The figure shows three views and two pictorial views of one solid part (mm, origin at its lowest corner). Answer the questions. Give positions to 0.01 mm unless a question says otherwise; leave off trailing zeros. Loops run counter-clockwise (first coordinate to the right, second up) from the corner with the lowest first, then second, coordinate; pieces in that order, holes last. Notation, with made-up numbers: M 64,-37 L 72,-37 A22 ccw 72,-11 Z; hole C -4,86.5 d5. An arc over 180 degrees is marked long. Answer in a Markdown table with one row per item. Add a question column.
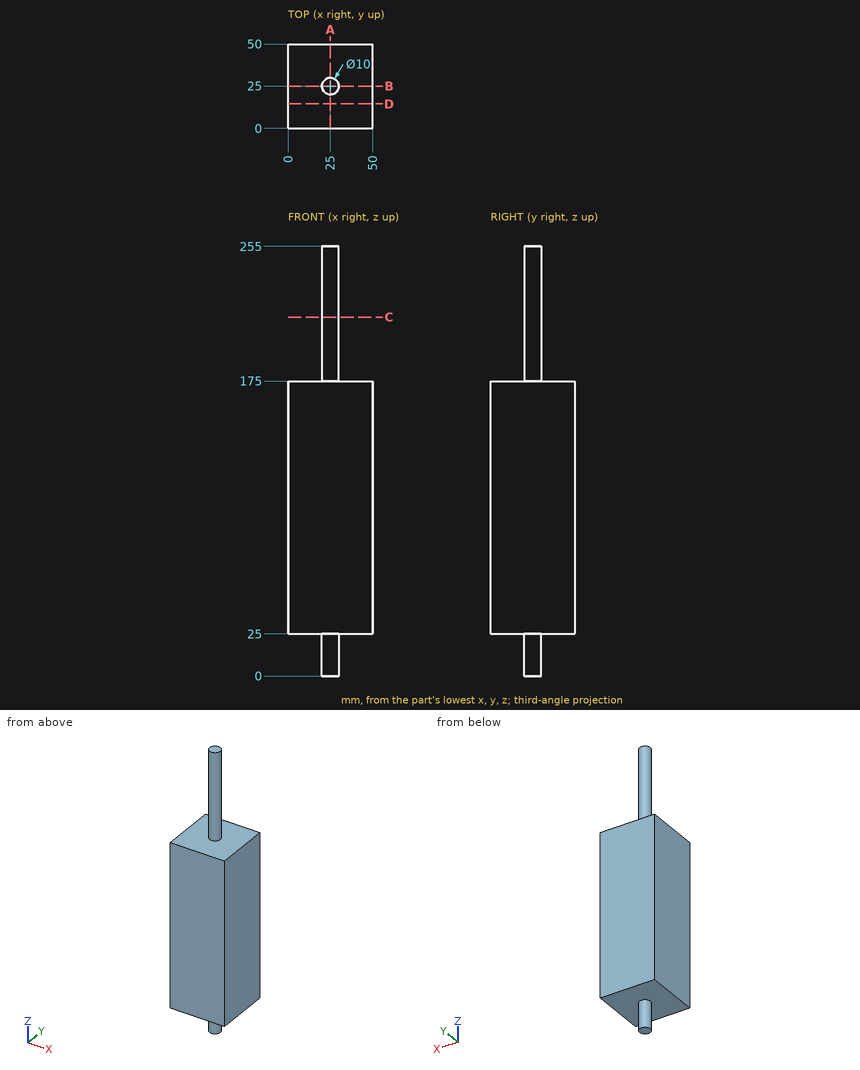
(1) Section A-A, the plane x = 25 is taken. Determine the outline of the cut face in (y, z).
(2) Section D-D, the plane y = 14.5 is taken. Determine the outline of the cut face in (x, z).
(3) Each of these flat-tipped pins is pushed along its axis until it touches: P1, Ø4, axis at x = 9.5, y = 37.5, coming from the +Z side; P2, Ø6, axis at x = 25.5, y = 16, coming from the -Z side. Where does it stop, or does it pass through?
(4) Section C-C, the plane z = 213 is taken. Determine the outline of the cut face in (x, y).
(5) Consider line 1 along Z through (x, y) = (19.5, 45.5); line 2 along Y through (x, z) = (21, 224); line 3 along X through (y, z) = (27.5, 222.5). Determine where each line is inside the solid, lowest interval first. Write a range as from..to.
Numbers:
| question | item | result |
|---|---|---|
| 1 | outline | M 0,25 L 20,25 L 20,0 L 30,0 L 30,25 L 50,25 L 50,175 L 30,175 L 30,255 L 20,255 L 20,175 L 0,175 Z |
| 2 | outline | M 0,25 L 50,25 L 50,175 L 0,175 Z |
| 3 | P1 | stops at z = 175 |
| 3 | P2 | stops at z = 25 |
| 4 | outline | C 25,25 d10 |
| 5 | line 1 | z = 25..175 |
| 5 | line 2 | y = 22..28 |
| 5 | line 3 | x = 20.67..29.33 |
